Check sheet for the modelled part. Datum: model origin and axes. Units: mm. A direction names the side the tool comes from. Coordinates: 2 decimals unless noted, no trailing zeros. Loops run counter-clockwise (first coordinate to the right, second up) from the corner with the lowest first, then second, coordinate; pieces in that order, holes last. Notation, with made-up numbers: M 42,84 L 95,84 A20 cw 95,104 Z; hole C 60,53 d11. An arc over 180 degrees is marked long. Answer in a Markdown table with one row per item. Add a question column.
```python
from build123d import *

# Parameters (mm, degrees)
SKETCH1_R           = 11.495405
BOSS_EXTRUDE2_DEPTH = 4.7625
BOSS_EXTRUDE3_DEPTH = 3.175
FILLET1_R           = 1.5875


with BuildPart() as part:
    # Sketch1 → Boss-Extrude2 (new, symmetric)
    with BuildSketch(Plane.XY):
        with BuildLine():
            ThreePointArc((14.672983865, 0.491098707), (-4.158599684, 14.079903484), (-12.585193267, -7.559797873))
            ThreePointArc((-12.585193267, -7.559797873), (4.158599684, -14.079903484), (14.672983865, 0.491098707))
        make_face()
        with Locations(Location((0, 0, 0), (0, 0, 180))):
            Circle(SKETCH1_R, mode=Mode.SUBTRACT)
    extrude(amount=BOSS_EXTRUDE2_DEPTH, both=True)

    # Sketch1_4 → Boss-Extrude3 (add, symmetric)
    with BuildSketch(Plane.XY):
        with BuildLine():
            ThreePointArc((-12.585193267, -7.559797873), (-10.89585042, -11.492870345), (-10.31875, -15.734319794))
            Line((-10.31875, -15.734319794), (-10.31875, -49.389319794))
            Line((-10.31875, -49.389319794), (10.31875, -49.389319794))
            Line((10.31875, -49.389319794), (10.31875, -34.936520731))
            Line((10.31875, -34.936520731), (21.966281014, -52.934138627))
            Line((21.966281014, -52.934138627), (39.292025986, -41.721424085))
            Line((39.292025986, -41.721424085), (17.211603503, -7.603033986))
            ThreePointArc((17.211603503, -7.603033986), (15.391641433, -3.728672569), (14.672983865, 0.491098707))
            ThreePointArc((14.672983865, 0.491098707), (4.158599684, -14.079903484), (-12.585193267, -7.559797873))
        make_face()
        with BuildLine():
            ThreePointArc((5.55625, -39.070569794), (0, -44.626819794), (-5.55625, -39.070569794))
            Line((-5.55625, -39.070569794), (-5.55625, -27.958069794))
            ThreePointArc((-5.55625, -27.958069794), (0, -22.401819794), (5.55625, -27.958069794))
            Line((5.55625, -27.958069794), (5.55625, -39.070569794))
        make_face(mode=Mode.SUBTRACT)
        with BuildLine():
            ThreePointArc((29.687419875, -35.646101109), (28.04160399, -43.329532516), (20.358172583, -41.683716631))
            Line((20.358172583, -41.683716631), (14.32055706, -32.354469339))
            ThreePointArc((14.32055706, -32.354469339), (15.966372945, -24.671037931), (23.649804353, -26.316853816))
            Line((23.649804353, -26.316853816), (29.687419875, -35.646101109))
        make_face(mode=Mode.SUBTRACT)
    extrude(amount=BOSS_EXTRUDE3_DEPTH, both=True)

    # Fillet1
    fillet1_edges = [part.edges().sort_by_distance(p)[0] for p in [
        (-10.31875, -49.389319794, 0),
        (10.31875, -49.389319794, 0),
        (10.31875, -34.936520731, 0),
        (21.966281014, -52.934138627, 0),
        (39.292025986, -41.721424085, 0),
    ]]
    fillet(fillet1_edges, radius=FILLET1_R)


solid = part.part
```
Q1. Cross-section at D-D (x = 19). Record the cut outline in (y, z) (3 decimals).
Q2. Go/stop test with flat-tipped pins: pin 1 (5 mm diameter, centred on x = -0.5, z = -1, fed in from -Y); pin 2 (5 mm diameter, centred on y = -33, z = 1, fed in from -X); pin 3 (5 mm diameter, centred on y = -34.5, z = -1.5, fed in from +X); pin 4 (18.5 mm diameter, centred on x = 0, y = 0, fed in from -Z). Record where each tip stops, or that it passes through.
Q3. Thickness scan on L1, parallel to Y at x = 0, z = -2; L2, parallel to X at y = 9, z = 0.75; L3, parallel to Z at x = 16, y = -39 (3 decimals). Record the ranges inside material, lowest first.
Q4. Access from +Z, -Z, +X, -X, +Y, -Y to the whole of each face (thin tool, end or side, straight path). Record for faces 5 (the face through (-0.122, -22.403, 0.044)), 6 (the face through (-10.319, -32, 0)), 7 (the face through (17.116, -45.44, 0.044)).
Q5. Cross-section at C-C (x = 7). Record the cut outline in (y, z) (1 decimal).
Q6. Cross-section at B-B (z = -1.25). Count the separate pieces of the cut face and the enclosed holes in it, plus the area to 3 significant figures.
Q7. Mould release check, pull along X, two halves, no side actions. Record for faces 1 (the face through (-9.87, -48.91, 0.04)), 2 (the face through (5.556, -33, 0)), 3 (the face through (15.86, -24.74, 0.04)), 4 (the face through (-9, -8, -4.762)): released by +X, released by -X, zero draft, split by the parting line, or undercut.
Q8. Cross-section at A-A (x = 0). Record the cut outline in (y, z) (1 decimal), plus the area to 3 significant figures.
Answer key:
| question | item | result |
|---|---|---|
| 1 | outline | M -48.351,-3.175 L -39.585,-3.175 L -39.585,3.175 L -48.351,3.175 Z; M -23.779,-3.175 L -10.366,-3.175 L -10.366,3.175 L -23.779,3.175 Z |
| 2 | pin 1 | y = -49.39 |
| 2 | pin 2 | x = -10.32 |
| 2 | pin 3 | x = 36.24 |
| 2 | pin 4 | through |
| 3 | L1 | -49.39 to -44.63, -22.4 to -11.5, 11.5 to 14.68 |
| 3 | L2 | -11.6 to -7.15, 7.15 to 11.6 |
| 3 | L3 | -3.175 to 3.175 |
| 4 | face 5 | +Z, -Z |
| 4 | face 6 | +Z, -Z, -X, -Y |
| 4 | face 7 | +Z, -Z, -Y |
| 5 | outline | M -49.4,-3.2 L -12.9,-3.2 L -12.9,-4.8 L -9.1,-4.8 L -9.1,4.8 L -12.9,4.8 L -12.9,3.2 L -49.4,3.2 Z; M 9.1,-4.8 L 12.9,-4.8 L 12.9,4.8 L 9.1,4.8 Z |
| 6 | separate pieces | 1 |
| 6 | enclosed holes | 3 |
| 6 | area | 1,310 mm^2 |
| 7 | face 1 | released by -X |
| 7 | face 2 | undercut |
| 7 | face 3 | undercut |
| 7 | face 4 | zero draft |
| 8 | outline | M -49.4,-3.2 L -44.6,-3.2 L -44.6,3.2 L -49.4,3.2 Z; M -22.4,-3.2 L -14.7,-3.2 L -14.7,-4.8 L -11.5,-4.8 L -11.5,4.8 L -14.7,4.8 L -14.7,3.2 L -22.4,3.2 Z; M 11.5,-4.8 L 14.7,-4.8 L 14.7,4.8 L 11.5,4.8 Z |
| 8 | area | 140 mm^2 |
